Geometry check sheet. Reference: drawing and pictorial views, mm from the part's lowest x, y, z. A direction names the side the tool comes from. Give positions to 0.01 mm unless a question says otherwise; leave off trailing zeros. Loops run counter-clockwise (first coordinate to the right, second up) from the corner with the lowest first, then second, coordinate; pieces in that order, holes last. Notation, with made-up numbers: (-36.75, -31.75) - (14.25, -31.75) arc R17 ccw to (14.25, -17.75) - close; hole circle Ø5 at (33.5, -30). An arc over 180 degrees is marked (long way). Put each result on its own line as item: value. Start each with the question number.
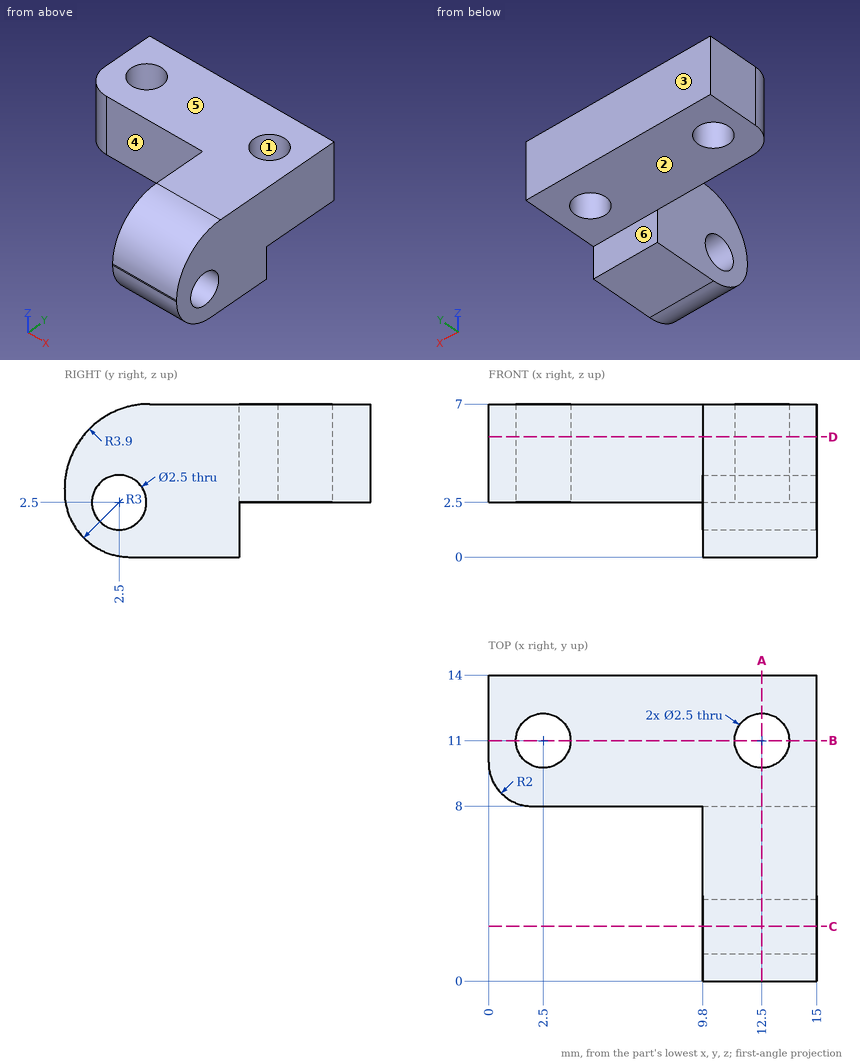
1) Depth check by flat-ended pin: P1, Ø3, axis at x = 2.5, y = 11, coming from the -Z side; P2, Ø2, axis at y = 3, z = 2.5, coming from the -X side. Enter the tip coordinate at first touch or a pass-through.
2) Scan lines: line 1 along X through (y, z) = (11.25, 3.25); line 2 along Y through (x, z) = (2.5, 5); line 3 along X through (y, z) = (5.5, 2). Record each from-to range of solid material in increasing order. Write a range as from..to.
3) Section check B-B, the plane y = 11. Enter the section's corners in (x, z).
4) Set-up check for the marked faces 4, 5 and 6: record each of +Z, -Z, +X, -X, +Y, -Y from which the full face is reachable in a straight line by a thin tool's end or side.
5) Section check C-C, the plane y = 2.5. Enter the section's corners in (x, z), plus the area to 3 significant figures.
6) Section check A-A, the plane x = 12.5. Enter the section's corners in (y, z), plus the area to 3 significant figures.
7) Section check D-D, the plane z = 5.5. Enter the section's corners in (x, y).
8) Draft check along Y on the marked faces 1, 2 and 3. Enter one of: pulls with the +Y half, pulls with the -Y half, needs draft (parallel to the pull), parting line crosses it, or undercut.
Results are:
1. P1: stops at z = 2.5
1. P2: stops at x = 9.8
2. line 1: x = 0..1.28, 3.72..11.28, 13.72..15
2. line 2: y = 8..9.75, 12.25..14
2. line 3: x = 9.8..15
3. outline: (0, 2.5) - (1.25, 2.5) - (1.25, 7) - (0, 7) - close; (3.75, 2.5) - (11.25, 2.5) - (11.25, 7) - (3.75, 7) - close; (13.75, 2.5) - (15, 2.5) - (15, 7) - (13.75, 7) - close
4. face 4: +Z, -Z, -X, -Y
4. face 5: +Z, +X, -X, +Y, -Y
4. face 6: -Z, +X, -X, +Y
5. outline: (9.8, 0.04) - (15, 0.04) - (15, 1.25) - (9.8, 1.25) - close; (9.8, 3.75) - (15, 3.75) - (15, 6.74) - (9.8, 6.74) - close
5. area: 21.8 mm2
6. outline: (0, 3) arc R3 ccw to (3, 0) - (8, 0) - (8, 2.5) - (9.75, 2.5) - (9.75, 7) - (3.9, 7) arc R3.9 ccw to (0, 3.1) - close; (12.25, 2.5) - (14, 2.5) - (14, 7) - (12.25, 7) - close; hole circle Ø2.5 at (2.5, 2.5)
6. area: 61.6 mm2
7. outline: (0, 10) arc R2 ccw to (2, 8) - (9.8, 8) - (9.8, 0.83) - (15, 0.83) - (15, 14) - (0, 14) - close; hole circle Ø2.5 at (2.5, 11); hole circle Ø2.5 at (12.5, 11)
8. face 1: undercut
8. face 2: needs draft
8. face 3: pulls with the +Y half
